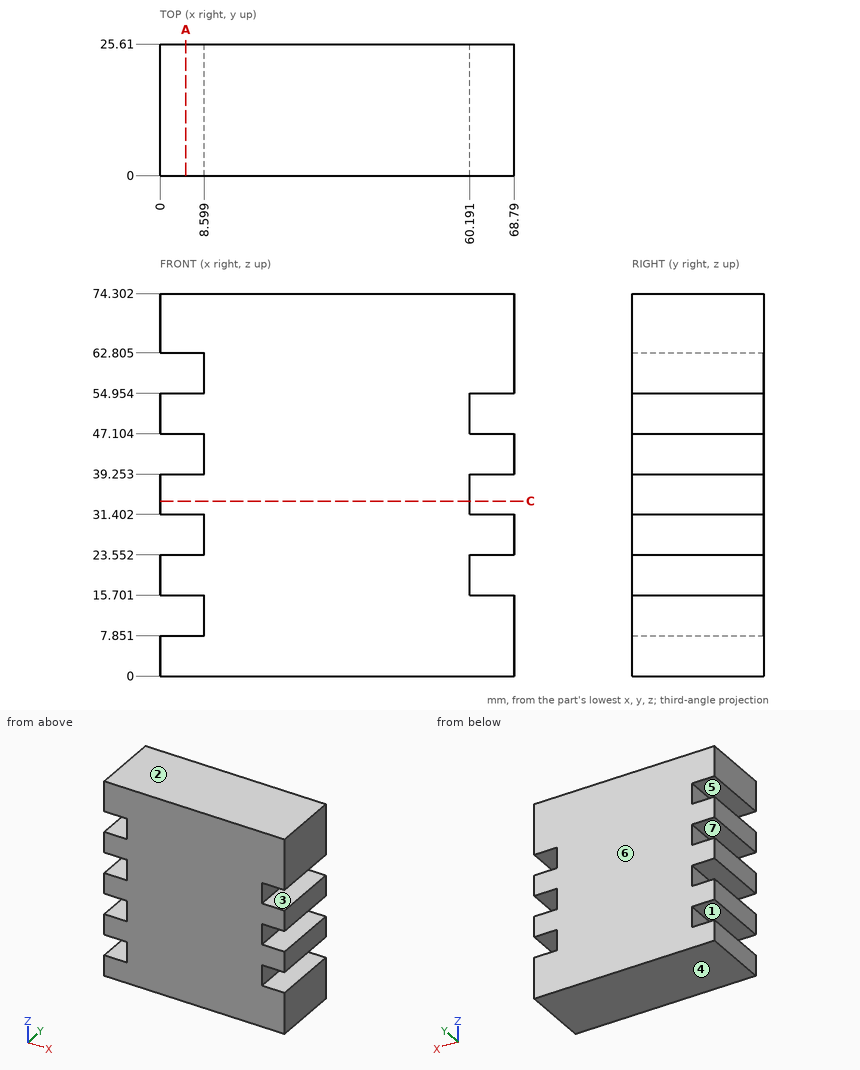
Source: three-view drawing plus pictorial views. Frame: mm from the lowest corner of the part. A direction names the side the tool comes from. Round coordinates to 2 decimals unless told otherwise and drop trailing zeros. Loops run counter-clockwise (first coordinate to the right, second up) from the corner with the lowest first, then second, coordinate; pieces in that order, holes last.
1. Mould query, pull axis Z, two halves, no side actions, for the marked faces 4, 5, 6 and 7. Classes: released by +Z, released by -Z, zero draft, split by the parting line, or undercut.
2. Ray query, L1, parallel to Z at x = 64, y = 9.5 (1 decimal); L2, parallel to X at y = 21.25, z = 25; L3, parallel to X at y = 13.25, z = 22.5. Return the intervals inside material, ascending.
3. Section query A-A on x = 5. Give the number of separate pieces and of enclosed holes in the cut face, and give its area (3 significant figures).
4. Contact query for flat-ended pins moving along their axis: pin 1 (4 mm diameter, centred on y = 15.5, z = 61, fed in from -X); pin 2 (2.5 mm diameter, centred on y = 10.5, z = 36, fed in from +X). Output: stop coordinate, or through.
5. Section query C-C on z = 34. Output: boundary loops of the cut face in (x, y), and give its area (3 significant figures).
6. Access query for the marked faces 1, 2 and 3. Directions: +Z, -Z, +X, -X, +Y, -Y. A direction counts if a zero-diameter tool reaches every point of the face in a straight line with its end or side. Return the directions, or none.
Answers below:
1. face 4: released by -Z
1. face 5: undercut
1. face 6: zero draft
1. face 7: undercut
2. L1: z = 0 to 15.7, 23.6 to 31.4, 39.3 to 47.1, 55 to 74.3
2. L2: x = 8.6 to 68.79
2. L3: x = 0 to 60.19
3. separate pieces: 5
3. enclosed holes: 0
3. area: 1,100 mm2
4. pin 1: stops at x = 0
4. pin 2: stops at x = 60.19
5. outline: (0, 0) - (60.19, 0) - (60.19, 25.61) - (0, 25.61) - close
5. area: 1,540 mm2
6. face 1: -X, +Y, -Y
6. face 2: +Z, +X, -X, +Y, -Y
6. face 3: +X, +Y, -Y
